from build123d import *

# Parameters (mm, degrees)
BOSS_EXTRUDE1_DEPTH = 3
CUT_EXTRUDE1_REACH  = 5
SKETCH3_R           = 8


with BuildPart() as part:
    # Sketch2 → Boss-Extrude1 (new body)
    with BuildSketch(Plane(origin=(0, 0, 0), x_dir=(0, 0, -1), z_dir=(1, 0, 0))):
        Polygon((8.679494794, 7.615753637), (-2.255688722, 11.324539802), (-10.935183515, 3.708786165), (-8.679494794, -7.615753637), (2.255688722, -11.324539802), (10.935183515, -3.708786165), align=None)
    extrude(amount=BOSS_EXTRUDE1_DEPTH)

    # Sketch3 → Cut-Extrude1 (cut, up to next)
    with BuildSketch(Plane.ZY, mode=Mode.PRIVATE) as cut_extrude1_sk1:
        Circle(SKETCH3_R)
    cut_extrude1_tool1 = extrude(cut_extrude1_sk1.sketch, amount=-CUT_EXTRUDE1_REACH, mode=Mode.PRIVATE) & part.part
    add(cut_extrude1_tool1.solids().sort_by_distance((0, 0, 0))[0], mode=Mode.SUBTRACT)


solid = part.part
Build history of the part. All positions in model axes, mm. Give positions to 0.01 mm unless a question says otherwise; leave off trailing zeros. Order: outer loops, then holes, each group sorted by start corner. A loop starts at its lowest first (then second) coordinate and runs counter-clockwise, first axis right, second up. Notation, with made-up numbers: M -8,-35 L 10,-35 A12 cw 10,-28 Z; hole C 15,56 d3. An arc over 180 degrees is marked long. Put each result on its own line as item: value.
Item 1: Cut at C-C on y = 1.5. Write the cut outline in (x, z), then the cut area to 3 significant figures.
Results are:
outline: M 0,-9.9 L 3,-9.9 L 3,-7.86 L 0,-7.86 Z; M 0,7.86 L 3,7.86 L 3,10.5 L 0,10.5 Z
area: 14.0 mm2
Item 2: Cut at B-B on z = -3. Write the cut outline in (x, y).
Results are:
outline: M 0,-10.67 L 3,-10.67 L 3,-7.42 L 0,-7.42 Z; M 0,7.42 L 3,7.42 L 3,9.54 L 0,9.54 Z
Item 3: Pull direction Y, two halves, no side cores. Call faces 1 (the face through (3, 8, -3)), 2 (the face through (1.479, -1.874, 9.823)), 3 (the face through (1.479, 1.874, -9.823)), 4 (the face through (1.48, -7.81, -1.73)): +Y half, -Y half, draft (parallel to the pull), parting line (faces both ways), or undercut.
Results are:
face 1: draft
face 2: -Y half
face 3: +Y half
face 4: undercut
Item 4: Cut at A-A on x = 1.2. Write the cut outline in (y, z).
Results are:
outline: M -11.32,-2.26 L -3.71,-10.94 L 7.62,-8.68 L 11.32,2.26 L 3.71,10.94 L -7.62,8.68 Z; hole C 0,0 d16
Item 5: Wall check: probe 1 along Y at (x, z) = (1.65, -5.75); probe 2 along Y at (x, z) = (2.15, 3); probe 3 along Z at (x, y) = (1.05, 1.75). Give the ranges that are in metal, low to high.
Results are:
probe 1: -8.26 to -5.56, 5.56 to 8.61
probe 2: -9.54 to -7.42, 7.42 to 10.67
probe 3: -9.85 to -7.81, 7.81 to 10.55
Item 6: Cut at D-D on y = 8.5. Write the cut outline in (x, z), then the cut area to 3 significant figures.
Results are:
outline: M 0,-6.07 L 3,-6.07 L 3,5.47 L 0,5.47 Z
area: 34.6 mm2
Item 7: Drop flat-ended pins along their axis: pin 1 Ø1 at (x, y) = (2.5, -4.5) entering from -Z; pin 2 Ø1 at (x, z) = (2.5, -2.5) entering from +Y; pin 3 Ø1 at (x, y) = (1, 1.5) entering from -Z; pin 4 Ø10 at (y, z) = (-1.5, 2) entering from +X. Give the stop position or say it passes through.
Results are:
pin 1: z = -10.6
pin 2: y = 9.88
pin 3: z = -10
pin 4: through
